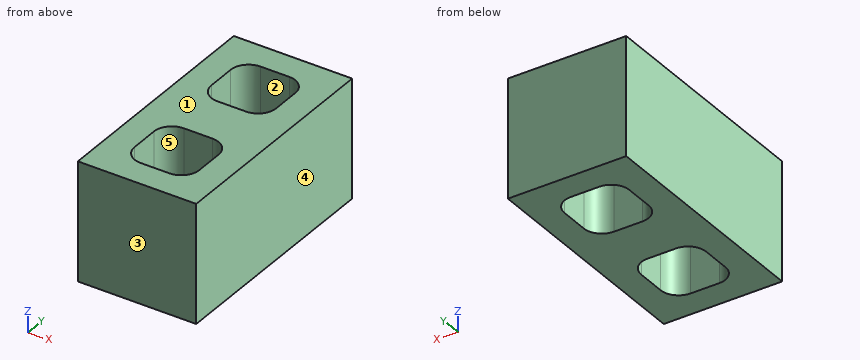
from build123d import *

# Parameters (mm, degrees)
F0_W     = 16.764
F0_H     = 33.02
F1_DEPTH = 8.382
F2_W     = 9.144
F2_H     = 9.144
F3_DEPTH = 25.4
F4_R     = 2.54


# Not quite as in the source:
# - two fillets or chamfers of one size are made in one step
# - a pattern or mirror of a feature is missing from the dataset's text; its kind, count and spacing are read off the source's solid


with BuildPart() as f1:
    # F0 (on Top) → F1 (new body, symmetric)
    with BuildSketch(Plane.XY):
        Rectangle(F0_W, F0_H)
    extrude(amount=F1_DEPTH, both=True)

    # F2 (on face) → F3 (cut)
    with BuildSketch(Plane.XY.offset(8.382)):
        with Locations((0, 8.128)):
            Rectangle(F2_W, F2_H)
    f3 = extrude(amount=-F3_DEPTH, mode=Mode.SUBTRACT)

    # F3_copies: F3 across plane
    add(f3.mirror(Plane(origin=(0, 0, 0), x_dir=(0, 0, -1), z_dir=(0, -1, 0))), mode=Mode.SUBTRACT)

    # F4
    f4_edges = [f1.edges().sort_by_distance(p)[0] for p in [
        (-4.572, 12.7, 0),
        (4.572, 12.7, 0),
        (-4.572, 3.556, 0),
        (-4.572, -12.7, 0),
        (4.572, -12.7, 0),
        (4.572, -3.556, 0),
        (-4.572, -3.556, 0),
        (4.572, 3.556, 0),
    ]]
    fillet(f4_edges, radius=F4_R)


solid = f1.part
Geometry: final body of the model. Coordinates: model frame, mm. Face numbers are marked on the shaded views. A direction names the side the tool comes from. Coordinates: 2 decimals unless noted, no trailing zeros. Write each loop counter-clockwise with the first axis right and the second up, starting at its lowest first coordinate (ties: lowest second). Pieces come first, ordered by that corner, then holes. Notation, with made-up numbers: (-34, 11) - (12, 11) arc R10 ccw to (12, 23) - close; hole circle Ø3 at (47, 44.25). An arc over 180 degrees is marked (long way). Return JSON: item names as keys, results as strings.
Item 1: Section query C-C (z = 7.25). Output: boundary loops of the cut face in (x, y).
Completed:
{"outline": "(-8.38, -16.51) - (8.38, -16.51) - (8.38, 16.51) - (-8.38, 16.51) - close; hole (-4.57, -10.16) arc R2.54 ccw to (-2.03, -12.7) - (2.03, -12.7) arc R2.54 ccw to (4.57, -10.16) - (4.57, -6.1) arc R2.54 ccw to (2.03, -3.56) - (-2.03, -3.56) arc R2.54 ccw to (-4.57, -6.1) - close; hole (-4.57, 6.1) arc R2.54 ccw to (-2.03, 3.56) - (2.03, 3.56) arc R2.54 ccw to (4.57, 6.1) - (4.57, 10.16) arc R2.54 ccw to (2.03, 12.7) - (-2.03, 12.7) arc R2.54 ccw to (-4.57, 10.16) - close"}
Item 2: Section query A-A (y = 7.5). Output: boundary loops of the cut face in (x, z), and give its area (3 significant figures).
Completed:
{"outline": "(-8.38, -8.38) - (-4.57, -8.38) - (-4.57, 8.38) - (-8.38, 8.38) - close; (4.57, -8.38) - (8.38, -8.38) - (8.38, 8.38) - (4.57, 8.38) - close", "area": "128 mm2"}
Item 3: Reachability of the marked faces 1 and 2 from +Z, -Z, +X, -X, +Y, -Y: full face, straight path, thin tool, end or side. Return the list, or none.
Completed:
{"face 1": "+Z, +X, -X, +Y, -Y", "face 2": "+Z, -Z"}
Item 4: Line query: L1, parallel to X at y = -9.5, z = -7; L2, parallel to Y at x = 0.75, z = -4; L3, parallel to Y at x = -3.75, z = -6.5. Output: solid intervals per line, ascending.
Completed:
{"L1": "x = -8.38 to -4.57, 4.57 to 8.38", "L2": "y = -16.51 to -12.7, -3.56 to 3.56, 12.7 to 16.51", "L3": "y = -16.51 to -12.03, -4.23 to 4.23, 12.03 to 16.51"}
Item 5: Section query B-B (x = 3.5). Output: boundary loops of the cut face in (y, z).
Completed:
{"outline": "(-16.51, -8.38) - (-12.23, -8.38) - (-12.23, 8.38) - (-16.51, 8.38) - close; (-4.02, -8.38) - (4.02, -8.38) - (4.02, 8.38) - (-4.02, 8.38) - close; (12.23, -8.38) - (16.51, -8.38) - (16.51, 8.38) - (12.23, 8.38) - close"}
Item 6: Section query D-D (y = -4.5). Output: boundary loops of the cut face in (x, z).
Completed:
{"outline": "(-8.38, -8.38) - (-4.01, -8.38) - (-4.01, 8.38) - (-8.38, 8.38) - close; (4.01, -8.38) - (8.38, -8.38) - (8.38, 8.38) - (4.01, 8.38) - close"}
Item 7: Pull-direction query (X, two-part tool) for the marked faces 3, 4 and 5; classes: +X half, -X half, draft (parallel to the pull), parting line (faces both ways), or undercut.
Completed:
{"face 3": "draft", "face 4": "+X half", "face 5": "undercut"}
